Read the model definition and answer for the solid it produces. Units are mm, in the model's axes. A direction names the side the tool comes from. Round coordinates to 2 decimals unless told otherwise and drop trailing zeros. Order: outer loops, then holes, each group sorted by start corner. A loop starts at its lowest first (then second) coordinate and runs counter-clockwise, first axis right, second up. Notation, with made-up numbers: (13.25, -36.5) -> (29.25, -36.5) arc R12 cw to (29.25, -14.5) -> close; hole circle Ø9 at (51.5, 67.5). An arc over 180 degrees is marked (long way). Use a Markdown table: item, result. Add a question column.
1. Given pin 1 (1.6 mm diameter, centred on x = 5.5, z = 5.5, fed in from +Y); pin 2 (0.8 mm diameter, centred on x = 5.5, z = 5, fed in from -Y); pin 3 (0.7 mm diameter, centred on x = 7, z = -0.5, fed in from -Y), each flat-ended and moving along its own axis, determine where each tip first touches the part or whether it passes through.
2. For faces 1 (the face through (4.8, 3, 5)), 2 (the face through (6, 1.8, 5)), 3 (the face through (6.3, 3, 5)), 4 (the face through (6, 3.3, 5)), determine the directions among +Z, -Z, +X, -X, +Y, -Y from which every point of the face is accessible in a straight line to the end or side of a thin tool.
3. Section D-D, the plane z = 0.75 is taken. Give the vertices of the cut face in (x, y), then the cut area to 4 significant figures.
4. Section C-C, the plane z = 1.75 is taken. Give the vertices of the cut face in (x, y), then the cut area to 4 significant figures.
5. Section A-A, the plane y = 2.1 is taken. Give the vertices of the cut face in (x, z), then the cut area to 4 significant figures.
6. Section B-B, the plane x = 1.15 is taken. Give the vertices of the cut face in (y, z), then the cut area to 3 significant figures.
7. Consider L1, parallel to Y at x = 6, z = 2.25; L2, parallel to X at y = 3.05, z = 4.75. Determine where each line is inside the solid, lowest interval first. Write a range as [from, to].
```python
from build123d import *

# Parameters (mm, degrees)
SKETCH_1_W                 = 9.1
SKETCH_1_H                 = 3.5
EXTRUDE_1_DEPTH            = 3.5
SKETCH_2_W                 = 1.5
SKETCH_2_H                 = 1.5
EXTRUDE_2_DEPTH            = 4
SKETCH_3_R                 = 0.35
EXTRUDE_3_DEPTH            = 0.5
SKETCH_5_W                 = 0.6
SKETCH_5_H                 = 0.3
PATTERN_LINEAR_1_COUNT     = 2
PATTERN_LINEAR_1_PITCH     = 2.5
PATTERN_LINEAR_1_COL_COUNT = 2
PATTERN_LINEAR_1_COL_PITCH = 2.5


with BuildPart() as part:
    # 草图1 → 凸台-拉伸1 (new body)
    with BuildSketch(Plane.XY):
        with Locations((4.55, 1.75)):
            Rectangle(SKETCH_1_W, SKETCH_1_H)
    extrude(amount=EXTRUDE_1_DEPTH)

    # 草图2 → 凸台-拉伸2 (add)
    with BuildSketch(Plane.XY.offset(3.5)):
        with Locations((5.55, 2.55)):
            Rectangle(SKETCH_2_W, SKETCH_2_H)
    extrude(amount=EXTRUDE_2_DEPTH)

    # 草图3 → 凸台-拉伸3 (add)
    with BuildSketch(Plane.XZ):
        with Locations(Location((1.15, 1.75, 0), (0, 0, 90))):
            Circle(SKETCH_3_R)
        with Locations(Location((7.95, 1.75, 0), (0, 0, 90))):
            Circle(SKETCH_3_R)
    extrude(amount=EXTRUDE_3_DEPTH)

    # 扫描1: sweep along a path in 草图4
    with BuildLine(Plane.ZY.offset(-4.55)) as sweep_1_path:
        Line((-2.2, 0.15), (-1.060798769, 0.15))
        Line((-1.060798769, 0.15), (-0.708229264, 0.608340356))
        Line((-0.708229264, 0.608340356), (0, 0.608340356))
    # 草图5 → 扫描1 (sweep)
    with BuildSketch(Plane(origin=(0, 0, -2.2), x_dir=(-1, 0, 0), z_dir=(0, 0, -1))):
        with Locations((-4.55, 0.15)):
            Rectangle(SKETCH_5_W, SKETCH_5_H)
    sweep_1 = sweep(path=sweep_1_path.line, transition=Transition.RIGHT)

    # 阵列(线性)1: 扫描1 ×2
    with Locations(*[(i * PATTERN_LINEAR_1_PITCH, 0, 0) for i in range(1, PATTERN_LINEAR_1_COUNT)]):
        add(sweep_1)

    # 阵列(线性)1 col: 扫描1 ×2
    with Locations(*[(-i * PATTERN_LINEAR_1_COL_PITCH, 0, 0) for i in range(1, PATTERN_LINEAR_1_COL_COUNT)]):
        add(sweep_1)


solid = part.part
```
Verdict:
| question | item | result |
|---|---|---|
| 1 | pin 1 | stops at y = 3.3 |
| 1 | pin 2 | stops at y = 1.8 |
| 1 | pin 3 | stops at y = 0.18 |
| 2 | face 1 | +Z, -X, +Y, -Y |
| 2 | face 2 | +Z, +X, -X, -Y |
| 2 | face 3 | +Z, +X, +Y, -Y |
| 2 | face 4 | +Z, +X, -X, +Y |
| 3 | outline | (0, 0) -> (9.1, 0) -> (9.1, 3.5) -> (0, 3.5) -> close |
| 3 | area | 31.85 mm2 |
| 4 | outline | (0, 0) -> (0.8, 0) -> (0.8, -0.5) -> (1.5, -0.5) -> (1.5, 0) -> (7.6, 0) -> (7.6, -0.5) -> (8.3, -0.5) -> (8.3, 0) -> (9.1, 0) -> (9.1, 3.5) -> (0, 3.5) -> close |
| 4 | area | 32.55 mm2 |
| 5 | outline | (0, 0) -> (9.1, 0) -> (9.1, 3.5) -> (6.3, 3.5) -> (6.3, 7.5) -> (4.8, 7.5) -> (4.8, 3.5) -> (0, 3.5) -> close |
| 5 | area | 37.85 mm2 |
| 6 | outline | (-0.5, 1.4) -> (0, 1.4) -> (0, 0) -> (3.5, 0) -> (3.5, 3.5) -> (0, 3.5) -> (0, 2.1) -> (-0.5, 2.1) -> close |
| 6 | area | 12.6 mm2 |
| 7 | L1 | y = [0, 3.5] |
| 7 | L2 | x = [4.8, 6.3] |
